```python
from build123d import *

# Parameters (mm, degrees)
SKETCH1_R                                       = 2.5
BOSS_EXTRUDE1_DEPTH                             = 5
BOSS_EXTRUDE1_2_DEPTH                           = 5
BOSS_EXTRUDE1_3_DEPTH                           = 5
BOSS_EXTRUDE1_4_DEPTH                           = 5
SKETCH3_W                                       = 77.6
SKETCH3_H                                       = 61.3
BOSS_EXTRUDE2_DEPTH                             = 3
SKETCH4_W                                       = 77.6
SKETCH4_H                                       = 61.3
SKETCH4_W_2                                     = 73.6
SKETCH4_H_2                                     = 57.3
BOSS_EXTRUDE3_DEPTH                             = 17
CUT_EXTRUDE2_REACH                              = 86.292
SKETCH5_W                                       = 13.5
SKETCH5_H                                       = 11
SKETCH5_W_2                                     = 10.5
FILLET1_R                                       = 1
FILLET2_R                                       = 1
SKETCH7_W                                       = 75.2
SKETCH7_H                                       = 58.9
CUT_EXTRUDE3_DEPTH                              = 2
SKETCH2_R                                       = 1
CUT_EXTRUDE1_DEPTH                              = 52.647482998
CSK_FOR_M2_FLAT_HEAD_MACHINE_SCREW1_D           = 2.4
CSK_FOR_M2_FLAT_HEAD_MACHINE_SCREW1_CSINK_D     = 4.4
CSK_FOR_M2_FLAT_HEAD_MACHINE_SCREW1_CSINK_ANGLE = 90


with BuildPart() as part:
    # Sketch1 → Boss-Extrude1 (new body)
    with BuildSketch(Plane(origin=(0, 0, 0), x_dir=(1, 0, 0), z_dir=(0, 1, 0))):
        with Locations(Location((-32.6, 19.09, 0), (0, 0, 270))):
            Circle(SKETCH1_R)
    extrude(amount=-BOSS_EXTRUDE1_DEPTH)



with BuildPart() as body_2:
    # Sketch1 → Boss-Extrude1 2 (new body)
    with BuildSketch(Plane(origin=(0, 0, 0), x_dir=(1, 0, 0), z_dir=(0, 1, 0))):
        with Locations(Location((-32.6, -8.85, 0), (0, 0, 270))):
            Circle(SKETCH1_R)
    extrude(amount=-BOSS_EXTRUDE1_2_DEPTH)


with BuildPart() as body_3:
    # Sketch1 → Boss-Extrude1 3 (new body)
    with BuildSketch(Plane(origin=(0, 0, 0), x_dir=(1, 0, 0), z_dir=(0, 1, 0))):
        with Locations(Location((19.8, 24.15, 0), (0, 0, 270))):
            Circle(SKETCH1_R)
    extrude(amount=-BOSS_EXTRUDE1_3_DEPTH)


with BuildPart() as body_4:
    # Sketch1 → Boss-Extrude1 4 (new body)
    with BuildSketch(Plane(origin=(0, 0, 0), x_dir=(1, 0, 0), z_dir=(0, 1, 0))):
        with Locations(Location((18.5, -24.05, 0), (0, 0, 270))):
            Circle(SKETCH1_R)
    extrude(amount=-BOSS_EXTRUDE1_4_DEPTH)


with BuildPart() as part_1:
    add(part.part)

    add(body_2.part)  # Boss-Extrude2 merges body 2

    add(body_3.part)  # Boss-Extrude2 merges body 3

    add(body_4.part)  # Boss-Extrude2 merges body 4
    # Sketch3 → Boss-Extrude2 (add)
    with BuildSketch(Plane.XZ.offset(5)):
        with Locations((-1, 0)):
            Rectangle(SKETCH3_W, SKETCH3_H)
    extrude(amount=BOSS_EXTRUDE2_DEPTH)

    # Sketch4 → Boss-Extrude3 (add)
    with BuildSketch(Plane(origin=(0, -5, 0), x_dir=(1, 0, 0), z_dir=(0, 1, 0))):
        with Locations((-1, 0)):
            Rectangle(SKETCH4_W, SKETCH4_H)
        with Locations((-1, 0)):
            Rectangle(SKETCH4_W_2, SKETCH4_H_2, mode=Mode.SUBTRACT)
    extrude(amount=BOSS_EXTRUDE3_DEPTH)

    # Sketch5 → Cut-Extrude2 (cut, up to next)
    with BuildSketch(Plane(origin=(37.8, 0, 0), x_dir=(0, 0, -1), z_dir=(1, 0, 0)), mode=Mode.PRIVATE) as cut_extrude2_sk1:
        with Locations((-11.45, 6.5)):
            Rectangle(SKETCH5_W, SKETCH5_H)
    cut_extrude2_tool1 = extrude(cut_extrude2_sk1.sketch, amount=-CUT_EXTRUDE2_REACH, mode=Mode.PRIVATE) & part_1.part
    # Sketch5 → Cut-Extrude2 (cut, up to next)
    with BuildSketch(Plane(origin=(37.8, 0, 0), x_dir=(0, 0, -1), z_dir=(1, 0, 0)), mode=Mode.PRIVATE) as cut_extrude2_sk2:
        with Locations((18.4, 6.5)):
            Rectangle(SKETCH5_W_2, SKETCH5_H)
    cut_extrude2_tool2 = extrude(cut_extrude2_sk2.sketch, amount=-CUT_EXTRUDE2_REACH, mode=Mode.PRIVATE) & part_1.part
    add(cut_extrude2_tool1.solids().sort_by_distance((37.8, 6.5, 11.45))[0], mode=Mode.SUBTRACT)
    add(cut_extrude2_tool2.solids().sort_by_distance((37.8, 6.5, -18.4))[0], mode=Mode.SUBTRACT)

    # Fillet1
    fillet1_edges = [part_1.edges().sort_by_distance(p)[0] for p in [
        (-1, -5, 28.65),
        (-1, -5, -28.65),
        (-37.8, -5, 0),
        (35.8, 3.5, -28.65),
        (-37.8, 3.5, -28.65),
        (-37.8, 3.5, 28.65),
        (35.8, 3.5, 28.65),
        (37.8, -8, 0),
    ]]
    fillet(fillet1_edges, radius=FILLET1_R)

    # Fillet2
    fillet2_edges = [part_1.edges().sort_by_distance(p)[0] for p in [
        (-39.8, 2, 30.65),
        (-39.8, 2, -30.65),
        (-39.8, -8, 0),
        (-1.5, -8, -30.65),
        (-1.5, -8, 30.65),
        (37.8, 2.5, 30.65),
        (37.507106781, -7.707106781, 30.65),
        (37.8, 2.5, -30.65),
        (37.507106781, -7.707106781, -30.65),
    ]]
    fillet(fillet2_edges, radius=FILLET2_R)

    # Sketch7 → Cut-Extrude3 (cut)
    with BuildSketch(Plane(origin=(0, 12, 0), x_dir=(1, 0, 0), z_dir=(0, 1, 0))):
        with Locations((-1, 0)):
            Rectangle(SKETCH7_W, SKETCH7_H)
    extrude(amount=-CUT_EXTRUDE3_DEPTH, mode=Mode.SUBTRACT)

    # Sketch2 → Cut-Extrude1 (cut, through all)
    with BuildSketch(Plane(origin=(0, 0, 0), x_dir=(1, 0, 0), z_dir=(0, 1, 0))):
        with Locations(Location((-32.6, -8.85, 0), (0, 0, 270))):
            Circle(SKETCH2_R)
        with Locations(Location((-32.6, 19.09, 0), (0, 0, 270))):
            Circle(SKETCH2_R)
        with Locations(Location((19.8, 24.15, 0), (0, 0, 270))):
            Circle(SKETCH2_R)
        with Locations(Location((18.5, -24.05, 0), (0, 0, 270))):
            Circle(SKETCH2_R)
    extrude(amount=-CUT_EXTRUDE1_DEPTH, mode=Mode.SUBTRACT)

    # CSK for M2 Flat Head Machine Screw1 (through all)
    with Locations(Plane(origin=(0, -8, 0), x_dir=(-1, 0, 0), z_dir=(0, -1, 0))):
        with Locations((32.6, 19.09), (32.6, -8.85), (-18.5, -24.05), (-19.8, 24.15)):
            CounterSinkHole(CSK_FOR_M2_FLAT_HEAD_MACHINE_SCREW1_D / 2, CSK_FOR_M2_FLAT_HEAD_MACHINE_SCREW1_CSINK_D / 2, counter_sink_angle=CSK_FOR_M2_FLAT_HEAD_MACHINE_SCREW1_CSINK_ANGLE)


solid = part_1.part
```
Here's how the part is built. I have some questions about the finished solid (model axes, mm). A direction names the side the tool comes from. Coordinates: 2 decimals unless noted, no trailing zeros. Order: outer loops, then holes, each group sorted by start corner. A loop starts at its lowest first (then second) coordinate and runs counter-clockwise, first axis right, second up.
Item 1: If we section it at D-D, the plane z = -14.5: List the corners of the cut face in (x, y) for me, then the cut area to 3 significant figures.
Response values:
outline: (-39.8, -7) arc R1 ccw to (-38.8, -8) - (36.8, -8) arc R1 ccw to (37.8, -7) - (37.8, 1) - (35.8, 1) - (35.8, -5) - (-36.8, -5) arc R1 cw to (-37.8, -4) - (-37.8, 10) - (-38.6, 10) - (-38.6, 12) - (-39.8, 12) - close
area: 277 mm2
Item 2: Which directions (+Z, -Z, +X, -X, +Y, -Y) give clear straight access to the entire face, cutting with the end or side of a thin tool? Please do faces 1 (the face through (-30.49, -2.46, -17.75)), 2 (the face through (37, 6, -23.65)), 3 (the face through (37.8, 2, 0)).
Response values:
face 1: +Y
face 2: +X, +Y
face 3: +Z, -Z, +X, +Y, -Y
Item 3: Thinking about a two-plate mould opening in X: for faces 4 (the face through (37, 1, -18)), 5 (the face through (-39.8, 2, 0)), 6 (the face through (-34, 0, 8)), which applies, pulls with the +X half, pulls with the -X half, needs draft (parallel to the pull), parting line crosses it, or undercut?
Response values:
face 4: needs draft
face 5: pulls with the -X half
face 6: undercut
Item 4: I need wall thicknesses on probe 1 along X at (y, z) = (-2, 8.85); probe 2 along Z at (x, y) = (27, 9.5); probe 3 along Z at (x, y) = (-34.5, -4.5). Which ranges of each line are inside material? Lowest first, please.
Response values:
probe 1: x = -39.8 to -37.8, -35.1 to -33.8, -31.4 to -30.1, 35.8 to 37.8
probe 2: z = -30.65 to -28.65, 28.65 to 30.65
probe 3: z = -30.65 to -28.52, -20.71 to -17.47, 7.23 to 10.47, 28.52 to 30.65
Item 5: If we section it at A-A, the plane z = 24.05: List the corners of the cut face in (x, y) for me.
Response values:
outline: (-39.8, -7) arc R1 ccw to (-38.8, -8) - (16.3, -8) - (17.3, -7) - (17.3, 0) - (16, 0) - (16, -5) - (-36.8, -5) arc R1 cw to (-37.8, -4) - (-37.8, 10) - (-38.6, 10) - (-38.6, 12) - (-39.8, 12) - close; (19.7, -7) - (20.7, -8) - (36.8, -8) arc R1 ccw to (37.8, -7) - (37.8, 12) - (36.6, 12) - (36.6, 10) - (35.8, 10) - (35.8, -5) - (21, -5) - (21, 0) - (19.7, 0) - close
Item 6: If we section it at B-B, the plane y = 4.75: List the corners of the cut face in (x, z) for me, then the cut area to 3 significant figures.
Response values:
outline: (-39.8, -29.65) arc R1 ccw to (-38.8, -30.65) - (36.8, -30.65) arc R1 ccw to (37.8, -29.65) - (37.8, -23.65) - (35.8, -23.65) - (35.8, -27.65) arc R1 cw to (34.8, -28.65) - (-36.8, -28.65) arc R1 cw to (-37.8, -27.65) - (-37.8, 27.65) arc R1 cw to (-36.8, 28.65) - (34.8, 28.65) arc R1 cw to (35.8, 27.65) - (35.8, 18.2) - (37.8, 18.2) - (37.8, 29.65) arc R1 ccw to (36.8, 30.65) - (-38.8, 30.65) arc R1 ccw to (-39.8, 29.65) - close; (35.8, -13.15) - (37.8, -13.15) - (37.8, 4.7) - (35.8, 4.7) - close
area: 492 mm2
Item 7: If we section it at C-C, the plane x = -6.5: List the corners of the cut face in (y, z) for me, then the cut area to 3 significant figures.
Response values:
outline: (-8, -29.65) arc R1 ccw to (-7, -30.65) - (12, -30.65) - (12, -29.45) - (10, -29.45) - (10, -28.65) - (-4, -28.65) arc R1 cw to (-5, -27.65) - (-5, 27.65) arc R1 cw to (-4, 28.65) - (10, 28.65) - (10, 29.45) - (12, 29.45) - (12, 30.65) - (-7, 30.65) arc R1 ccw to (-8, 29.65) - close
area: 249 mm2
Item 8: I'm going to push flat-ended pins straight in: pin 1 Ø8 at (x, z) = (-29, -9) entering from +Y; pin 2 Ø1 at (x, y) = (37, 8.5) entering from +Z; pin 3 Ø5.5 at (x, z) = (-33.5, -20) entering from +Y; pin 4 Ø1.6 at (x, z) = (37, 10.5) entering from +Y. Where does each tip first touch, or does it pass through?
Response values:
pin 1: stops at y = -5
pin 2: stops at z = 30.65
pin 3: stops at y = 0
pin 4: stops at y = 1
